The listing builds one solid part. Answer for the finished solid, in the listing's coordinates (mm). Face numbers are marked on the shaded views. A direction names the side the tool comes from. Coordinates: 2 decimals unless noted, no trailing zeros. Loops run counter-clockwise (first coordinate to the right, second up) from the corner with the lowest first, then second, coordinate; pieces in that order, holes last. Notation, with made-up numbers: (65, -37.75) -> (115, -37.75) arc R18 cw to (115, -15.75) -> close; hole circle Ø2 at (66.5, 3). An arc over 180 degrees is marked (long way). Answer in a Markdown table with one row per item.
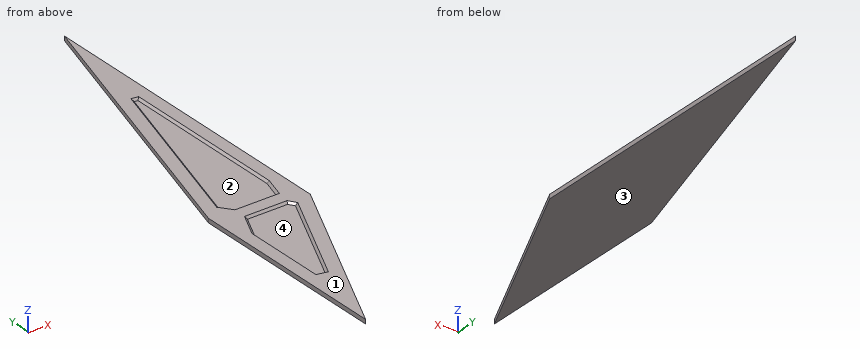
```python
from build123d import *

# Parameters (mm, degrees)
BOSS_EXTRU_1_DEPTH      = 10
ENL_V_MAT_EXTRU_1_DEPTH = 5
CHANFREIN1_SIZE         = 5


with BuildPart() as part:
    # Esquisse1 → Boss.-Extru.1 (new body)
    with BuildSketch(Plane.XY):
        Polygon((0, 0), (0, -450), (210, 0), (210, 727.857142857), (210, 769.998850412), (0, 42.141707555), align=None)
    extrude(amount=BOSS_EXTRU_1_DEPTH)

    # Esquisse2 → Enlèv. mat.-Extru.1 (cut)
    with BuildSketch(Plane.XY.offset(10)):
        Polygon((60, 37.900434867), (165.302631408, 37.900434867), (180, 88.841314442), (180, 497.798394051), (163.367347804, 500.149847834), (38.316326098, 66.724707975), align=None)
        Polygon((58.611734047, 6.655480102), (30, -54.655378569), (30, -254.773091326), (55.37312792, -260.402102926), (171.542290693, -11.468182697), (160, 6.655480102), align=None)
    extrude(amount=-ENL_V_MAT_EXTRU_1_DEPTH, mode=Mode.SUBTRACT)

    # Chanfrein1
    chanfrein1_edges = [part.edges().sort_by_distance(p)[0] for p in [
        (165.771145347, -2.406351297, 5),
        (113.457709307, -135.935142812, 5),
        (42.68656396, -257.587597126, 5),
        (30, -154.714234948, 5),
        (44.305867023, -23.999949233, 5),
        (109.305867023, 6.655480102, 5),
        (171.683673902, 498.974120942, 5),
        (180, 293.319854246, 5),
        (172.651315704, 63.370874655, 5),
        (112.651315704, 37.900434867, 5),
        (49.158163049, 52.312571421, 5),
        (100.841836951, 283.437277905, 5),
    ]]
    chamfer(chanfrein1_edges, length=CHANFREIN1_SIZE - 0.0001)  # a hair under: the kernel refuses the full size


solid = part.part
```
Item 1: A tool of negligible diameter and unlimited length cuts with its end or side. For the marked faces 1 and 2, from which of +Z, -Z, +X, -X, +Y, -Y can it reach the whole face along a straight path? Write none if from no direction.
Findings below:
| item | result |
|---|---|
| face 1 | +Z, +X, -X, +Y, -Y |
| face 2 | +Z |
Item 2: A cutting plane is placed at A-A, the plane z = 7.75. Determine the outline of the cut face in (x, y), plus the area to 3 significant figures.
Findings below:
| item | result |
|---|---|
| outline | (0, -450) -> (210, 0) -> (210, 770) -> (0, 42.14) -> close; hole (32.25, -252.97) -> (54.1, -257.81) -> (168.98, -11.64) -> (158.77, 4.41) -> (60.04, 4.41) -> (32.25, -55.15) -> close; hole (40.79, 67.18) -> (61.12, 40.15) -> (163.61, 40.15) -> (177.75, 89.16) -> (177.75, 495.84) -> (164.99, 497.65) -> close |
| area | 76,500 mm2 |
Item 3: A flat-ended cylindrical pin translates along its axis: pin 1 Ø1 at (x, z) = (179.5, 6.5) entering from -Y. Find the tip coordinate at first contact, or state that the pin passes through.
Findings below:
| item | result |
|---|---|
| pin 1 | stops at y = -66.43 |
Item 4: Determine the mould class of the marked faces 3 and 4 for opening direction Y: +Y half, -Y half, draft (parallel to the pull), parting line (faces both ways), or undercut.
Findings below:
| item | result |
|---|---|
| face 3 | draft |
| face 4 | undercut |
Item 5: Find the intervals of material crossed by probe 1 along X at (y, z) = (250.5, 1.5); probe 2 along X at (y, z) = (264, 7.25); probe 3 along X at (y, z) = (469.5, 8.75), in increasing order.
Findings below:
| item | result |
|---|---|
| probe 1 | x = 60.12 to 210 |
| probe 2 | x = 64.01 to 98.1, 177.25 to 210 |
| probe 3 | x = 123.3 to 155.83, 178.75 to 210 |
